Design review of the part built by this model. Coordinates are the model's own, in mm. Face numbers are marked on the shaded views. Round coordinates to 2 decimals unless told otherwise and drop trailing zeros. Write each loop counter-clockwise with the first axis right and the second up, starting at its lowest first coordinate (ties: lowest second). Pieces come first, ordered by that corner, then holes. Notation, with made-up numbers: (-25, 67) - (31, 67) arc R25 cw to (31, 82) - close; hole circle Ø2 at (-39, -35). An arc over 180 degrees is marked (long way). Use one line per item in the form item = value.
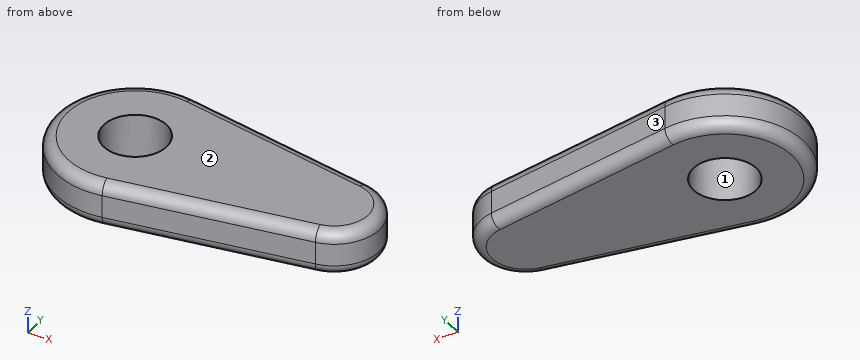
```python
from build123d import *

# Parameters (mm, degrees)
SKETCH_1_R      = 14
EXTRUDE_1_DEPTH = 20
FILLET_1_R      = 5
FILLET_2_R      = 5


with BuildPart() as part:
    # 草图1 → 凸台-拉伸1 (new body)
    with BuildSketch(Plane.XY):
        with BuildLine():
            Line((-32.661153615, 34.487793909), (52.782028203, 19.707310805))
            ThreePointArc((52.782028203, 19.707310805), (69.372937294, 0), (52.782028203, -19.707310805))
            Line((52.782028203, -19.707310805), (-32.661153615, -34.487793909))
            ThreePointArc((-32.661153615, -34.487793909), (-73.627062706, 0), (-32.661153615, 34.487793909))
        make_face()
        with Locations((-38.627062706, 0)):
            Circle(SKETCH_1_R, mode=Mode.SUBTRACT)
    extrude(amount=EXTRUDE_1_DEPTH)

    # 圆角1
    fillet_1_edges = [part.edges().sort_by_distance(p)[0] for p in [
        (-73.627062706, 0, 20),
        (10.060437294, -27.097552357, 20),
        (69.372937294, 0, 20),
        (10.060437294, 27.097552357, 20),
    ]]
    fillet(fillet_1_edges, radius=FILLET_1_R)

    # 圆角2
    fillet_2_edges = [part.edges().sort_by_distance(p)[0] for p in [
        (10.060437294, -27.097552357, 0),
        (-73.627062706, 0, 0),
        (10.060437294, 27.097552357, 0),
        (69.372937294, 0, 0),
    ]]
    fillet(fillet_2_edges, radius=FILLET_2_R)


solid = part.part
```
Q1. For P1, Ø1, axis at x = -43, z = 15, coming from the -Y side; P2, Ø8, axis at x = -26, z = 14.5, coming from the +Y side; P3, Ø2, axis at x = -4.5, z = 4.5, coming from the +Y side, all flat-tipped, find the tip position at first contact; note any pin that passes through.
Calculated:
P1 = -34.79
P2 = 34.03
P3 = 29.78
Q2. We need section A-A on y = 0. Write out the cut boundary in (x, z).
Calculated:
outline = (-73.63, 5) arc R5 ccw to (-68.63, 0) - (-52.63, 0) - (-52.63, 20) - (-68.63, 20) arc R5 ccw to (-73.63, 15) - close; (-24.63, 0) - (64.37, 0) arc R5 ccw to (69.37, 5) - (69.37, 15) arc R5 ccw to (64.37, 20) - (-24.63, 20) - close
Q3. To check wall thickness, follow line 1 along Y through (x, z) = (-39.5, 7); line 2 along X through (y, z) = (-10.5, 15.25); line 3 along Y through (x, z) = (-28, 5.75). State the ranges of each line that lie inside material, in increasing order. Write a range as from..to.
Calculated:
line_1 = -34.99..-13.97, 13.97..34.99
line_2 = -72.01..-47.89, -29.37..66.39
line_3 = -33.68..-9.11, 9.11..33.68
Q4. We need section B-B on z = 18.5. Write out the cut boundary in (x, y).
Calculated:
outline = (-32.9, -33.08) - (52.54, -18.3) arc R18.57 ccw to (52.54, 18.3) - (-32.9, 33.08) arc R33.57 ccw (long way) to start; hole circle Ø28 at (-38.63, 0)
Q5. Draft analysis for pull direction X (two halves, no side actions). For the marked faces 1, 2 and 3, state which applies: released by +X, released by -X, zero draft, split by the parting line, or undercut.
Calculated:
face_1 = undercut
face_2 = zero draft
face_3 = released by +X
